Verification items for the finished model (mm, model axes). A direction names the side the tool comes from. Give positions to 0.01 mm unless a question says otherwise; leave off trailing zeros. Loops run counter-clockwise (first coordinate to the right, second up) from the corner with the lowest first, then second, coordinate; pieces in that order, holes last. Notation, with made-up numbers: (-24, 31.5) -> (11, 31.5) arc R31 cw to (11, 64.5) -> close; hole circle Ø9 at (-37.5, 74). An arc over 180 degrees is marked (long way). Answer in a Markdown table with one row per item. Add a question column.
Q1. Section check B-B on x = -28.5. Enter the section's corners in (y, z).
Q2. Set-up check for faces 1 (the face through (-20.8, 31.4, 2.5)), 2 (the face through (-15, 21, 3)): record each of +Z, -Z, +X, -X, +Y, -Y from which the full face is reachable in a straight line by a thin tool's end or side.
Q3. Section check C-C on y = -23.5. Enter the section's corners in (x, z), and give its area (3 significant figures).
Q4. Release check for a two-part mould opening along Y. For faces 3 (the face through (-11.647, 9.484, 2.493)), 4 (the face through (-32.3, -1.76, 2.49)), 5 (the face through (-7, 42, 3)) record: pulls with the +Y half, pulls with the -Y half, needs draft (parallel to the pull), parting line crosses it, or undercut.
Q5. Material ranges on probe 1 along Y at (x, z) = (-28.5, 1); probe 2 along Y at (x, z) = (-7, 2.4); probe 3 along Z at (x, y) = (17.5, 19), recorded low to high.
Q6. Section check A-A on y = -41. Enter the section's corners in (x, z).
Q7. Gauge pin test, flat ends, axial feed: P1, Ø7, axis at x = -28.5, y = 41, coming from the -Z side; P2, Ø13, axis at x = -28.5, y = -41, coming from the +Z side. Record the tip position at first contact, or that the pin passes through.
```python
from build123d import *

# Parameters (mm, degrees)
F0_W     = 75
F0_H     = 100
F0_R     = 4
F1_DEPTH = 2
F2_R     = 1.523638
F2_R_2   = 1.567812
F2_R_3   = 1.559077
F2_R_4   = 1.322094
F2_R_5   = 1.567811
F2_R_6   = 1.402292
F2_R_7   = 1.701475
F2_R_8   = 1.652619
F2_R_9   = 1.523641
F2_R_10  = 1.884274
F2_R_11  = 1.652618
F2_R_12  = 1.685347
F2_R_13  = 1.411998
F2_R_14  = 1.478147
F2_R_15  = 1.478148
F2_R_16  = 1.523642
F2_R_17  = 1.725385
F2_R_18  = 1.411997
F2_R_19  = 1.332383
F2_R_20  = 1.927267
F2_R_21  = 1.869727
F2_R_22  = 1.421638
F2_R_23  = 1.756758
F2_R_24  = 1.627641
F2_R_25  = 1.49651
F2_R_26  = 1.660861
F2_R_27  = 1.66086
F2_R_28  = 1.421636
F2_R_29  = 1.559076
F2_R_30  = 1.478146
F2_R_31  = 1.587284
F2_R_32  = 1.332387
F2_R_33  = 1.487355
F2_R_34  = 1.660858
F2_R_35  = 1.652615
F2_R_36  = 1.81788
F3_DEPTH = 1
F4_W     = 28.54166
F4_H     = 14.979307
F5_DEPTH = 1


with BuildPart() as f1:
    # F0 (on Top) → F1 (new body)
    with BuildSketch(Plane.XY):
        Rectangle(F0_W, F0_H)
        with Locations((-28.5, -41)):
            Circle(F0_R, mode=Mode.SUBTRACT)
        with Locations((-28.5, 41)):
            Circle(F0_R, mode=Mode.SUBTRACT)
    extrude(amount=F1_DEPTH)

    # F2 (on face) → F3 (join)
    with BuildSketch(Plane.XY.offset(2)):
        with Locations((-33.796042, -8.345725)):
            Circle(F2_R)
        with Locations((-33.796042, -2.231038)):
            Circle(F2_R_2)
        with Locations((-33.796042, 3.553126)):
            Circle(F2_R_3)
        with Locations((-28.177142, -2.231038)):
            Circle(F2_R)
        with Locations((-21.236144, -2.231038)):
            Circle(F2_R_4)
        with Locations((-24.706643, 3.553126)):
            Circle(F2_R_5)
        with Locations((-15.782502, 3.553126)):
            Circle(F2_R_6)
        with Locations((-9.833077, 3.553126)):
            Circle(F2_R_7)
        with Locations((-4.875224, -2.231038)):
            Circle(F2_R_8)
        with Locations((0.578419, -2.231038)):
            Circle(F2_R_9)
        with Locations((-5.371009, -8.345725)):
            Circle(F2_R_10)
        with Locations((9.833081, -8.345725)):
            Circle(F2_R_11)
        with Locations((13.799365, -2.231038)):
            Circle(F2_R_12)
        with Locations((13.799365, 3.553126)):
            Circle(F2_R_3)
        with Locations((9.833081, 3.553126)):
            Circle(F2_R_6)
        with Locations((5.536273, 3.553126)):
            Circle(F2_R_13)
        with Locations((0.578419, 3.553126)):
            Circle(F2_R_14)
        with Locations((19.253004, 3.553126)):
            Circle(F2_R_15)
        with Locations((19.418268, -2.231038)):
            Circle(F2_R_16)
        with Locations((23.715075, 3.553126)):
            Circle(F2_R_17)
        with Locations((24.210861, -2.231038)):
            Circle(F2_R_18)
        with Locations((27.681356, -2.561562)):
            Circle(F2_R_19)
        with Locations((27.681356, -9.172035)):
            Circle(F2_R_20)
        with Locations((34.291834, -2.726824)):
            Circle(F2_R_21)
        with Locations((31.317115, 3.553126)):
            Circle(F2_R_6)
        with Locations((27.681356, 3.553126)):
            Circle(F2_R_22)
        with Locations((11.155175, 19.583523)):
            Circle(F2_R_23)
        with Locations((-6.693101, 21.401403)):
            Circle(F2_R_24)
        with Locations((-10.1636, 15.121453)):
            Circle(F2_R_25)
        with Locations((-10.328862, 10.494123)):
            Circle(F2_R_26)
        with Locations((-21.731928, 15.121453)):
            Circle(F2_R_3)
        with Locations((-15.121453, 21.070879)):
            Circle(F2_R_27)
        with Locations((-21.731928, 29.995019)):
            Circle(F2_R_12)
        with Locations((-21.731928, 36.27497)):
            Circle(F2_R)
        with Locations((-15.121453, 36.27497)):
            Circle(F2_R_28)
        with Locations((-15.121453, 41.89387)):
            Circle(F2_R_29)
        with Locations((-6.693101, 42.059135)):
            Circle(F2_R_30)
        with Locations((-6.693101, 36.27497)):
            Circle(F2_R)
        with Locations((0, 36.27497)):
            Circle(F2_R_31)
        with Locations((6.858371, 36.27497)):
            Circle(F2_R_32)
        with Locations((11.155175, 42.059135)):
            Circle(F2_R_33)
        with Locations((17.765649, 36.27497)):
            Circle(F2_R_34)
        with Locations((17.765649, 29.995019)):
            Circle(F2_R_35)
        with Locations((25.86348, 42.059135)):
            Circle(F2_R_36)
    extrude(amount=F3_DEPTH)

    # F4 (on face) → F5 (join)
    with BuildSketch(Plane.XY.offset(2)):
        with Locations((0, -29.250141)):
            Rectangle(F4_W, F4_H)
    extrude(amount=F5_DEPTH)


solid = f1.part
```
Taken from the geometry:
| question | item | result |
|---|---|---|
| 1 | outline | (-50, 0) -> (-45, 0) -> (-45, 2) -> (-50, 2) -> close; (-37, 0) -> (37, 0) -> (37, 2) -> (-0.74, 2) -> (-0.74, 3) -> (-3.72, 3) -> (-3.72, 2) -> (-37, 2) -> close; (45, 0) -> (50, 0) -> (50, 2) -> (45, 2) -> close |
| 2 | face 1 | +Z |
| 2 | face 2 | +Z, +X, -X, +Y, -Y |
| 3 | outline | (-37.5, 0) -> (37.5, 0) -> (37.5, 2) -> (14.27, 2) -> (14.27, 3) -> (-14.27, 3) -> (-14.27, 2) -> (-37.5, 2) -> close |
| 3 | area | 179 mm² |
| 4 | face 3 | undercut |
| 4 | face 4 | undercut |
| 4 | face 5 | needs draft |
| 5 | probe 1 | y = -50 to -45, -37 to 37, 45 to 50 |
| 5 | probe 2 | y = -36.74 to -21.76, -9.29 to -7.4, 19.8 to 23, 34.78 to 37.77, 40.61 to 43.51 |
| 5 | probe 3 | z = 0 to 2 |
| 6 | outline | (-37.5, 0) -> (-32.5, 0) -> (-32.5, 2) -> (-37.5, 2) -> close; (-24.5, 0) -> (37.5, 0) -> (37.5, 2) -> (-24.5, 2) -> close |
| 7 | P1 | passes through |
| 7 | P2 | stops at z = 2 |
